from build123d import *

# Parameters (mm, degrees)
SKETCH1_W           = 152.4
SKETCH1_H           = 127
BOSS_EXTRUDE1_DEPTH = 127
SKETCH2_W           = 50.8
SKETCH2_H           = 50.8
BOSS_EXTRUDE2_DEPTH = 25.4
SKETCH3_R           = 63.5
BOSS_EXTRUDE3_DEPTH = 25.4
SKETCH4_W           = 20.32
SKETCH4_H           = 20.32
BOSS_EXTRUDE4_DEPTH = 50.8
SKETCH5_W           = 152.4
SKETCH5_H           = 38.1
CUT_EXTRUDE1_DEPTH  = 253.726809025
SKETCH6_R           = 12.7
CUT_EXTRUDE2_DEPTH  = 209.682294409


with BuildPart() as part:
    # Sketch1 → Boss-Extrude1 (new body)
    with BuildSketch(Plane.XY):
        Rectangle(SKETCH1_W, SKETCH1_H)
    extrude(amount=BOSS_EXTRUDE1_DEPTH)

    # Sketch2 → Boss-Extrude2 (add)
    with BuildSketch(Plane.ZY.offset(76.2)):
        with Locations((63.5, 0)):
            Rectangle(SKETCH2_W, SKETCH2_H)
    extrude(amount=BOSS_EXTRUDE2_DEPTH)

    # Sketch3 → Boss-Extrude3 (add)
    with BuildSketch(Plane.ZY.offset(101.6)):
        with Locations((63.5, 0)):
            Circle(SKETCH3_R)
    extrude(amount=BOSS_EXTRUDE3_DEPTH)

    # Sketch4 → Boss-Extrude4 (add)
    with BuildSketch(Plane.ZY.offset(127)):
        with Locations((25.4, 0)):
            Rectangle(SKETCH4_W, SKETCH4_H)
        with Locations((101.6, 0)):
            Rectangle(SKETCH4_W, SKETCH4_H)
    extrude(amount=BOSS_EXTRUDE4_DEPTH)

    # Sketch5 → Cut-Extrude1 (cut, through all)
    with BuildSketch(Plane(origin=(0, 63.5, 0), x_dir=(1, 0, 0), z_dir=(0, 1, 0))):
        with Locations((0, -107.95)):
            Rectangle(SKETCH5_W, SKETCH5_H)
        with Locations((0, -19.05)):
            Rectangle(SKETCH5_W, SKETCH5_H)
    extrude(amount=-CUT_EXTRUDE1_DEPTH, mode=Mode.SUBTRACT)

    # Sketch6 → Cut-Extrude2 (cut, through all)
    with BuildSketch(Plane.XY.offset(88.9)):
        with Locations((12.7, 0)):
            Circle(SKETCH6_R)
    extrude(amount=-CUT_EXTRUDE2_DEPTH, mode=Mode.SUBTRACT)


solid = part.part
Build history of the part. All positions in model axes, mm. A direction names the side the tool comes from. Round coordinates to 2 decimals unless told otherwise and drop trailing zeros. Loops run counter-clockwise (first coordinate to the right, second up) from the corner with the lowest first, then second, coordinate; pieces in that order, holes last. Notation, with made-up numbers: (89, 39.25) -> (121, 39.25) arc R15 ccw to (121, 43.25) -> close; hole circle Ø7 at (83.5, 60.5). An arc over 180 degrees is marked (long way). Use CSV: the item, a comma, the result in double quotes. Start each with the question number.
Q1. Drill centre lines: L1, parallel to Y at x = 12.7, z = 74; L2, parallel to X at y = 56, z = 56; L3, parallel to Z at x = 2.5, y = -31. Where is each one in solid material? Low to high.
Q2. Saw through at B-B on y = 0. Give the cut face in (x, z).
Q3. Which spindle directions (+Z, -Z, +X, -X, +Y, -Y) get a long thin tool onto all of the face, cutting with end or side? Do faces 4 (the face through (-152, 10.16, 101)), 5 (the face through (-11, -1, 88.9)), 6 (the face through (-152, -10.16, 101)), 7 (the face through (-11, -1, 38.1)), 8 (the face through (-89, 25.4, 63)). Say none if no direction does.
Q4. Saw through at C-C on z = 63.5. Give the cut face in (x, y).
Q5. Saw through at D-D on x = -160. Give the cut face in (y, z).
Q6. Flat gauge pins, fed straight in: pin 1 Ø16.5 at (x, z) = (-159.5, 26.5) entering from -Y; pin 2 Ø6 at (x, z) = (-159.5, 98.5) entering from +Y; pin 3 Ø10 at (x, y) = (-145.5, 2.5) entering from +Z; pin 4 Ø15 at (x, y) = (12.7, 0) entering from +Z. Where does each tip first touch, or does it go through?
Q7. Mould opens along Z. For faces 1 (the face through (-89, -25.4, 63)), 2 (the face through (-152, 0, 91.44)), 3 (the face through (-152, 0, 15.24)) say: +Z half, -Z half, draft (parallel to the pull), parting line (faces both ways), or undercut.
Q8. Saw through at A-A on x = 12.7. Give the cut face in (y, z), and give its area (3 significant figures).
Solutions:
1,L1,"y = -63.5 to -12.7, 12.7 to 63.5"
1,L2,"x = -127 to -101.6, -76.2 to 76.2"
1,L3,"z = 38.1 to 88.9"
2,outline,"(-177.8, 15.24) -> (-127, 15.24) -> (-127, 0) -> (-101.6, 0) -> (-101.6, 38.1) -> (0, 38.1) -> (0, 88.9) -> (-101.6, 88.9) -> (-101.6, 127) -> (-127, 127) -> (-127, 111.76) -> (-177.8, 111.76) -> (-177.8, 91.44) -> (-127, 91.44) -> (-127, 35.56) -> (-177.8, 35.56) -> close; (25.4, 38.1) -> (76.2, 38.1) -> (76.2, 88.9) -> (25.4, 88.9) -> close"
3,face 4,"+Z, -Z, -X, +Y"
3,face 5,"+Z, +X, +Y, -Y"
3,face 6,"+Z, -Z, -X, -Y"
3,face 7,"-Z, +X, +Y, -Y"
3,face 8,"+Z, -Z, +Y"
4,outline,"(-127, -63.5) -> (-101.6, -63.5) -> (-101.6, -25.4) -> (-76.2, -25.4) -> (-76.2, -63.5) -> (76.2, -63.5) -> (76.2, 63.5) -> (-76.2, 63.5) -> (-76.2, 25.4) -> (-101.6, 25.4) -> (-101.6, 63.5) -> (-127, 63.5) -> close; hole circle Ø25.4 at (12.7, 0)"
5,outline,"(-10.16, 15.24) -> (10.16, 15.24) -> (10.16, 35.56) -> (-10.16, 35.56) -> close; (-10.16, 91.44) -> (10.16, 91.44) -> (10.16, 111.76) -> (-10.16, 111.76) -> close"
6,pin 1,"stops at y = -10.16"
6,pin 2,"stops at y = 10.16"
6,pin 3,"stops at z = 111.76"
6,pin 4,"passes through"
7,face 1,"draft"
7,face 2,"undercut"
7,face 3,"-Z half"
8,outline,"(-63.5, 38.1) -> (-12.7, 38.1) -> (-12.7, 88.9) -> (-63.5, 88.9) -> close; (12.7, 38.1) -> (63.5, 38.1) -> (63.5, 88.9) -> (12.7, 88.9) -> close"
8,area,"5,160 mm^2"
